from build123d import *

# Parameters (mm, degrees)
RESSALTO_EXTRUS_O3_DEPTH = 60
ESBO_O5_R                = 6
CORTE_EXTRUS_O1_DEPTH    = 17
ESBO_O7_W                = 30.866068748
ESBO_O7_H                = 32.5
ESBO_O7_H_2              = 7.5
CORTE_EXTRUS_O2_DEPTH    = 15
ESBO_O8_R                = 1
CORTE_EXTRUS_O3_DEPTH    = 5


with BuildPart() as part:
    # Esboço4 → Ressalto-extrusão3 (new body)
    with BuildSketch(Plane(origin=(0, 0, 0), x_dir=(1, 0, 0), z_dir=(0, 1, 0))):
        with BuildLine():
            Line((15.433034374, -3), (-15.433034374, -3))
            Line((-15.433034374, -3), (-15.433034374, 1))
            Line((-15.433034374, 1), (-7.433034374, 1))
            ThreePointArc((-7.433034374, 1), (0, 7.5), (7.433034374, 1))
            Line((7.433034374, 1), (15.433034374, 1))
            Line((15.433034374, 1), (15.433034374, -3))
        make_face()
    extrude(amount=RESSALTO_EXTRUS_O3_DEPTH)

    # Esboço5 → Corte-extrusão1 (cut)
    with BuildSketch(Plane(origin=(0, 0, 0), x_dir=(1, 0, 0), z_dir=(0, 1, 0))):
        Circle(ESBO_O5_R)
    extrude(amount=CORTE_EXTRUS_O1_DEPTH, mode=Mode.SUBTRACT)

    # Esboço6 → Corte-Revolução1 (revolve, cut)
    with BuildSketch(Plane.XY):
        Polygon((0, 17), (-5.75, 17), (-3.75, 70), (0, 70), align=None)
    revolve(axis=Axis((0, 70, 0), (0, -1, 0)), mode=Mode.SUBTRACT)

    # Esboço7 → Corte-extrusão2 (cut)
    with BuildSketch(Plane.XY.offset(3)):
        with Locations((0, 16.25)):
            Rectangle(ESBO_O7_W, ESBO_O7_H)
        with Locations((0, 56.25)):
            Rectangle(ESBO_O7_W, ESBO_O7_H_2)
    extrude(amount=-CORTE_EXTRUS_O2_DEPTH, mode=Mode.SUBTRACT)

    # Esboço8 → Corte-extrusão3 (cut, through all)
    with BuildSketch(Plane(origin=(0, 0, -1), x_dir=(-1, 0, 0), z_dir=(0, 0, -1))):
        with Locations((-10.433034374, 42.5)):
            Circle(ESBO_O8_R)
        with Locations((10.433034374, 42.5)):
            Circle(ESBO_O8_R)
    extrude(amount=-CORTE_EXTRUS_O3_DEPTH, mode=Mode.SUBTRACT)


solid = part.part
Input: part model. Units: mm. Frame: model coordinates. A direction names the side the tool comes from. Coordinates: 2 decimals unless noted, no trailing zeros. Write each loop counter-clockwise with the first axis right and the second up, starting at its lowest first coordinate (ties: lowest second). Pieces come first, ordered by that corner, then holes. Notation, with made-up numbers: M -34,42 L -1,42 A23 ccw -1,80 Z; hole C -17,-3 d4. An arc over 180 degrees is marked long. Answer as a JSON object with one key per item and string values. Group by question number.
(1) Set-up query: faces 1 (the face through (15.433, 42, 1)), 2 (the face through (-12, 42, -1)), 3 (the face through (12, 42, -1)). Return all of +Z, -Z, +X, -X, +Y, -Y with unobstructed straight access to the full face (end or side cutting, diameter ignored); none if empty.
(2) Section C-C on y = 37. Output: boundary loops of the cut face in (x, z), plus the area to 3 significant figures.
(3) Section B-B on y = 42.5. Output: boundary loops of the cut face in (x, z), plus the area to 3 significant figures.
(4) Mould query, pull axis X, two halves, no side actions, for faces 4 (the face through (-0.16, 42.64, -4.78)), 5 (the face through (-15.433, 42, 1)), 6 (the face through (9, 42, 3)). Classes: pulls with the +X half, pulls with the -X half, needs draft (parallel to the pull), parting line crosses it, or undercut.
(5) Ray query, line 1 along Z through (x, y) = (-12, 35.25); line 2 along X through (y, z) = (48.25, -2.25); line 3 along X through (y, z) = (37.25, -1.5). Return the intervals inside material, ascending. Write a range as [from, to].
(6) Section A-A on z = 0. Output: boundary loops of the cut face in (x, y), plus the area to 3 significant figures.
(7) Section D-D on x = 12. Output: boundary loops of the cut face in (y, z).
(8) Contact query for flat-ended pins moving along their axis: P1, Ø2.5, axis at x = -10.43, y = 42.5, coming from the -Z side; P2, Ø9, axis at x = 10.5, y = 47, coming from the -Z side; P3, Ø3, axis at x = 3.5, y = 46.5, coming from the -Z side. Output: stop coordinate, or through.
Result set:
{
 "1": {"face 1": "+Z, -Z, +X, +Y, -Y", "face 2": "-Z, -X, +Y, -Y", "face 3": "-Z, +X, +Y, -Y"},
 "2": {"outline": "M -15.43,-1 L -7.43,-1 A7.5 ccw 7.43,-1 L 15.43,-1 L 15.43,3 L 3.99,3 A5 cw long -3.99,3 L -15.43,3 Z", "area": "130 mm2"},
 "3": {"outline": "M -15.43,-1 L -11.43,-1 L -11.43,3 L -15.43,3 Z; M -9.43,-1 L -7.43,-1 A7.5 ccw 7.43,-1 L 9.43,-1 L 9.43,3 L 3.73,3 A4.79 cw long -3.73,3 L -9.43,3 Z; M 11.43,-1 L 15.43,-1 L 15.43,3 L 11.43,3 Z", "area": "118 mm2"},
 "4": {"face 4": "undercut", "face 5": "pulls with the -X half", "face 6": "needs draft"},
 "5": {"line 1": "z = [-1, 3]", "line 2": "x = [-7.15, -3.98], [3.98, 7.15]", "line 3": "x = [-7.35, -4.75], [4.75, 7.35]"},
 "6": {"outline": "M -15.43,32.5 L -5.17,32.5 L -4.41,52.5 L -15.43,52.5 Z; M 4.41,52.5 L 5.17,32.5 L 15.43,32.5 L 15.43,52.5 Z; hole C -10.43,42.5 d2; hole C 10.43,42.5 d2", "area": "420 mm2"},
 "7": {"outline": "M 32.5,-1 L 52.5,-1 L 52.5,3 L 32.5,3 Z"},
 "8": {"P1": "stops at z = -1", "P2": "stops at z = -4.5", "P3": "stops at z = -7.23"}
}
